The model under review builds one solid part; all positions refer to its coordinate system, in mm. Face numbers are marked on the shaded views. A direction names the side the tool comes from. Round coordinates to 2 decimals unless told otherwise and drop trailing zeros. Order: outer loops, then holes, each group sorted by start corner. A loop starts at its lowest first (then second) coordinate and runs counter-clockwise, first axis right, second up.
1) To check wall thickness, follow L1, parallel to X at y = 0.55, z = -7; L2, parallel to X at y = 1, z = -8.25; L3, parallel to X at y = 6, z = -12.25. State the ranges of each line that lie inside material, in increasing order.
2) Consider section D-D (z = -5). Give the boundary of the cut face in (x, y).
3) Consider section A-A (z = -7). Give the boundary of the cut face in (x, y), then the cut area to 3 significant figures.
4) Consider section B-B (x = -2.5). Give the boundary of the cut face in (y, z).
5) Machinability: for the marked faces 1 and 2, which of the approach directions +Z, -Z, +X, -X, +Y, -Y give a long, thin tool a straight path to every point of the face, cutting with its end or side? Answer none if there is none.
6) Consider section C-C (y = 3.5). Give the boundary of the cut face in (x, z), then the cut area to 3 significant figures.
7) Clearance check with flat-ended pins moving along their axes: P1, Ø2, axis at y = 5.5, z = -10.5, coming from the +X side; P2, Ø1.5, axis at x = 25, z = -6, coming from the +Y side; P3, Ø2.5, axis at x = -2.5, z = -7, coming from the +Y side; P4, Ø4, axis at y = 2, z = -1.5, coming from the -X side. State where each tip first meets the part, or that it passes through.
from build123d import *

# Parameters (mm, degrees)
SKETCH1_W           = 23
SKETCH1_H           = 14
BOSS_EXTRUDE1_DEPTH = 8.5
SKETCH2_W           = 33
SKETCH2_H           = 5
BOSS_EXTRUDE2_DEPTH = 1.2
SKETCH3_R           = 1.5
CUT_EXTRUDE1_DEPTH  = 10


with BuildPart() as part:
    # Sketch1 → Boss-Extrude1 (new body)
    with BuildSketch(Plane(origin=(0, 0, 0), x_dir=(1, 0, 0), z_dir=(0, 1, 0))):
        with Locations((11.5, 7)):
            Rectangle(SKETCH1_W, SKETCH1_H)
    extrude(amount=BOSS_EXTRUDE1_DEPTH)

    # Sketch2 → Boss-Extrude2 (add)
    with BuildSketch(Plane.XZ):
        with Locations((11.5, -7)):
            Rectangle(SKETCH2_W, SKETCH2_H)
    extrude(amount=-BOSS_EXTRUDE2_DEPTH)

    # Sketch3 → Cut-Extrude1 (cut)
    with BuildSketch(Plane(origin=(0, 1.2, 0), x_dir=(1, 0, 0), z_dir=(0, 1, 0))):
        with Locations(Location((-2.5, 7, 0), (0, 0, 270))):
            Circle(SKETCH3_R)
        with Locations(Location((25.5, 7, 0), (0, 0, 270))):
            Circle(SKETCH3_R)
    extrude(amount=-CUT_EXTRUDE1_DEPTH, mode=Mode.SUBTRACT)


solid = part.part
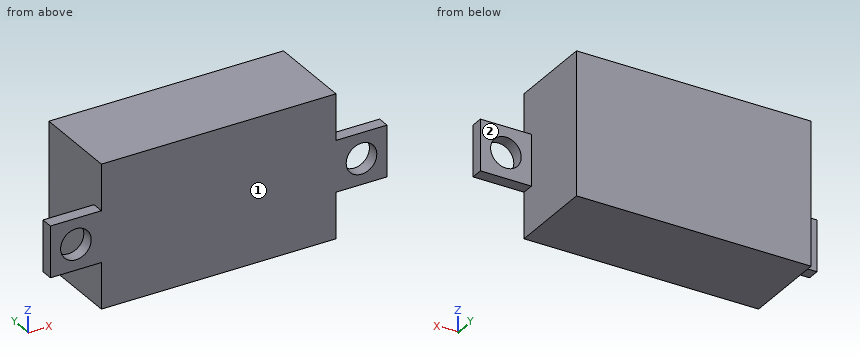
Answer below:
1. L1: x = -5 to -4, -1 to 24, 27 to 28
1. L2: x = -5 to -3.33, -1.67 to 24.67, 26.33 to 28
1. L3: x = 0 to 23
2. outline: (-5, 0) - (28, 0) - (28, 1.2) - (23, 1.2) - (23, 8.5) - (0, 8.5) - (0, 1.2) - (-5, 1.2) - close
3. outline: (-5, 0) - (-4, 0) - (-4, 1.2) - (-5, 1.2) - close; (-1, 0) - (24, 0) - (24, 1.2) - (23, 1.2) - (23, 8.5) - (0, 8.5) - (0, 1.2) - (-1, 1.2) - close; (27, 0) - (28, 0) - (28, 1.2) - (27, 1.2) - close
3. area: 200 mm2
4. outline: (0, -9.5) - (1.2, -9.5) - (1.2, -8.5) - (0, -8.5) - close; (0, -5.5) - (1.2, -5.5) - (1.2, -4.5) - (0, -4.5) - close
5. face 1: +Z, -Z, +X, -X, -Y
5. face 2: +Z, -Z, +X, +Y
6. outline: (0, -14) - (23, -14) - (23, 0) - (0, 0) - close
6. area: 322 mm2
7. P1: stops at x = 23
7. P2: stops at y = 1.2
7. P3: passes through
7. P4: stops at x = 0
